Could you check a few things on this drawing? It's one solid part, dimensions in mm from its lowest x, y, z. Give positions to 0.01 mm unless a question says otherwise; leave off trailing zeros. Loops run counter-clockwise (first coordinate to the right, second up) from the corner with the lowest first, then second, coordinate; pieces in that order, holes last. Notation, with made-up numbers: M 62,12 L 76,12 A26 ccw 76,46 Z; hole C 15.5,45 d11. An arc over 180 degrees is marked long. Answer as a JSON object with one key per item and string values.
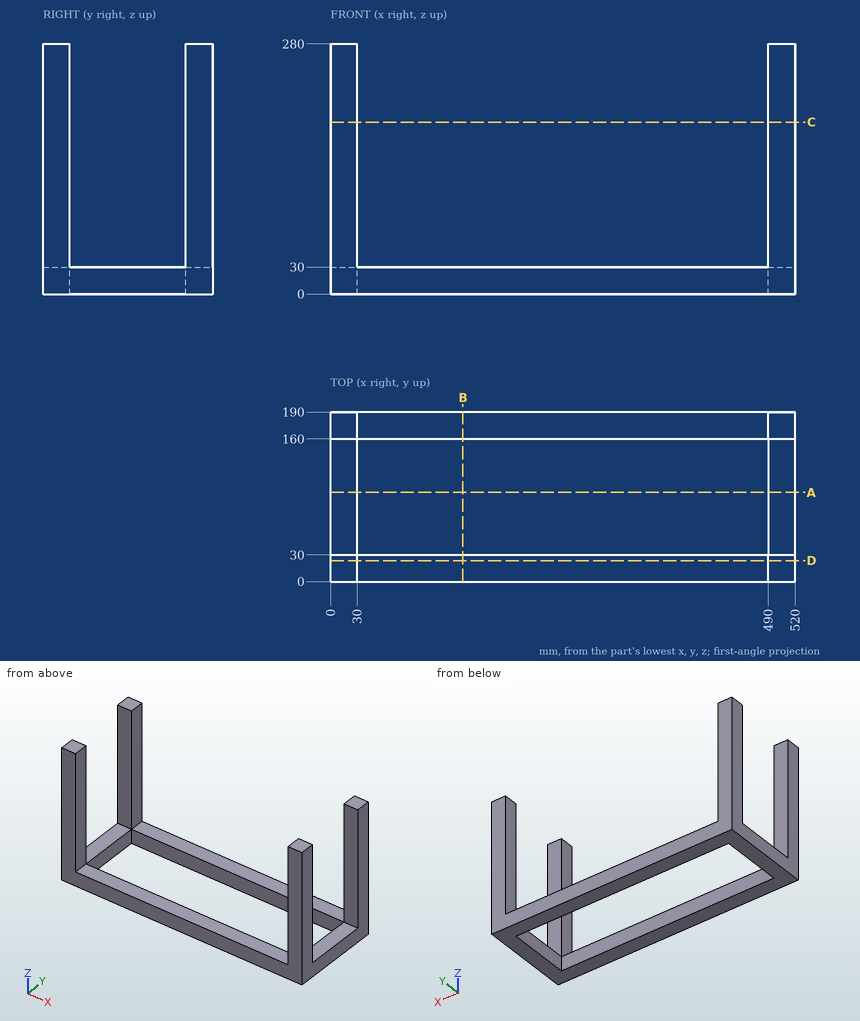
1) Will these pins go through, and if not, where does the flat tip stop? pin 1 Ø15 at (x, y) = (509, 119.5) entering from +Z; pin 2 Ø9 at (y, z) = (179.5, 116) entering from -X.
Answer list:
{"pin 1": "z = 30", "pin 2": "x = 0"}
2) Suppose I cut it at D-D, the plane y = 23.5. Write out the boundary of the cut face in (x, z).
Answer list:
{"outline": "M 0,0 L 520,0 L 520,280 L 490,280 L 490,30 L 30,30 L 30,280 L 0,280 Z"}
3) Suppose I cut it at C-C, the plane z = 192.5. Write out the boundary of the cut face in (x, y), and give its area (3 significant figures).
Answer list:
{"outline": "M 0,0 L 30,0 L 30,30 L 0,30 Z; M 0,160 L 30,160 L 30,190 L 0,190 Z; M 490,0 L 520,0 L 520,30 L 490,30 Z; M 490,160 L 520,160 L 520,190 L 490,190 Z", "area": "3,600 mm^2"}
4) Suppose I cut it at B-B, the plane x = 148. Write out the boundary of the cut face in (y, z).
Answer list:
{"outline": "M 0,0 L 30,0 L 30,30 L 0,30 Z; M 160,0 L 190,0 L 190,30 L 160,30 Z"}
5) Please list where these lines run through material, in increasing order: line 1 along X through (y, z) = (174, 76); line 2 along Y through (x, z) = (446.5, 11); line 3 along Z through (x, y) = (25.5, 47.5). Write a range as from..to.
Answer list:
{"line 1": "0..30, 490..520", "line 2": "0..30, 160..190", "line 3": "0..30"}
6) Suppose I cut it at A-A, the plane y = 100. Write out the boundary of the cut face in (x, z).
Answer list:
{"outline": "M 0,0 L 30,0 L 30,30 L 0,30 Z; M 490,0 L 520,0 L 520,30 L 490,30 Z"}
